```python
from build123d import *

# Parameters (mm, degrees)
F0_R      = 10
F1_DEPTH  = 10
F0_R_2    = 6
F2_DEPTH  = 20
F0_W      = 60
F0_H      = 20
F3_DEPTH  = 70
F4_R      = 16
F5_DEPTH  = 50
F6_R      = 3
F9_DEPTH  = 77.2
F10_DEPTH = 15
F11_DEPTH = 15


with BuildPart() as f1:
    # F0 (on Top) → F1 (new body)
    with BuildSketch(Plane.XY):
        with BuildLine():
            ThreePointArc((-5.564519, 60.884742), (-26.777723, 52.097945), (-35.564519, 30.884742))
            Line((-35.564519, 30.884742), (-35.564519, -9.115258))
            Line((-35.564519, -9.115258), (24.435481, -9.115258))
            Line((24.435481, -9.115258), (24.435481, 30.884742))
            ThreePointArc((24.435481, 30.884742), (15.648684, 52.097945), (-5.564519, 60.884742))
        make_face()
        with Locations((-5.564519, 30.884742)):
            Circle(F0_R, mode=Mode.SUBTRACT)
    extrude(amount=F1_DEPTH)

    # F0 (on Top) → F2 (join)
    with BuildSketch(Plane.XY):
        with Locations((-5.564519, 30.884742)):
            Circle(F0_R)
        with Locations((-5.564519, 30.884742)):
            Circle(F0_R_2, mode=Mode.SUBTRACT)
    extrude(amount=F2_DEPTH)

    # F0 (on Top) → F3 (join)
    with BuildSketch(Plane.XY):
        with Locations((-5.564519, -19.115258)):
            Rectangle(F0_W, F0_H)
    extrude(amount=F3_DEPTH)

    # F4 (on face) → F5 (join)
    with BuildSketch(Plane.XZ.offset(29.115258)):
        with Locations((-5.564519, 35)):
            Circle(F4_R)
    extrude(amount=F5_DEPTH)

    # F6
    f6_edges = [f1.edges().sort_by_distance(p)[0] for p in [
        (-21.564519, -79.115258, 35),
    ]]
    fillet(f6_edges, radius=F6_R)

    # F8 (on face) → F9 (cut)
    with BuildSketch(Plane(origin=(-35.564519, 0, 0), x_dir=(0, -1, 0), z_dir=(-1, 0, 0))):
        Polygon((19.833226, 70), (9.115258, 70), (9.115258, 30), align=None)
    extrude(amount=-F9_DEPTH, mode=Mode.SUBTRACT)

    # F8 (on face) → F10 (join)
    with BuildSketch(Plane(origin=(-35.564519, 0, 0), x_dir=(0, -1, 0), z_dir=(-1, 0, 0))):
        Polygon((19.833226, 70), (9.115258, 70), (9.115258, 30), align=None)
        Polygon((19.833226, 70), (9.115258, 30), (9.115258, 10), (-30.884742, 10), (-30.884742, 0), (29.115258, 0), (29.115258, 70), align=None)
    extrude(amount=-F10_DEPTH)

    # F7 (on face) → F11 (join)
    with BuildSketch(Plane.YZ.offset(24.435481)):
        Polygon((-9.115258, 10), (-9.115258, 30), (-19.833226, 70), (-29.115258, 70), (-29.115258, 0), (30.884742, 0), (30.884742, 10), align=None)
        Polygon((-9.115258, 30), (-9.115258, 70), (-19.833226, 70), align=None)
    extrude(amount=-F11_DEPTH)


solid = f1.part
```
Verification items for the finished model (mm, model axes). A direction names the side the tool comes from. Coordinates: 2 decimals unless noted, no trailing zeros. Order: outer loops, then holes, each group sorted by start corner. A loop starts at its lowest first (then second) coordinate and runs counter-clockwise, first axis right, second up. Notation, with made-up numbers: (63.25, 67) - (92.25, 67) arc R18 ccw to (92.25, 86) - close; hole circle Ø6 at (-27.75, 75). An arc over 180 degrees is marked (long way). Return JSON: item names as keys, results as strings.
(1) Section check B-B, the plane y = -44.5. Record the cut outline in (x, z).
Filled sheet:
{"outline": "circle Ø32 at (-5.56, 35)"}
(2) Section check A-A, the plane z = 53.5. Record the cut outline in (x, y).
Filled sheet:
{"outline": "(-35.56, -29.12) - (24.44, -29.12) - (24.44, -9.12) - (9.44, -9.12) - (9.44, -15.41) - (-20.56, -15.41) - (-20.56, -9.12) - (-35.56, -9.12) - close"}
(3) Section check C-C, the plane x = -26. Record the cut outline in (y, z).
Filled sheet:
{"outline": "(-29.12, 0) - (52.85, 0) - (52.85, 10) - (-9.12, 10) - (-9.12, 70) - (-29.12, 70) - close"}
(4) Mould release check, pull along X, two halves, no side actions. Record for faces 1 (the flat face through (-5.77, -14.4, 49.72)), 2 (the flat face through (-35.565, -12, 28)), 3 (the flat face through (-13, -29.115, 19)): pulls with the +X half, pulls with the -X half, needs draft (parallel to the pull), parting line crosses it, or undercut.
Filled sheet:
{"face 1": "undercut", "face 2": "pulls with the -X half", "face 3": "needs draft"}
(5) Access from +Z, -Z, +X, -X, +Y, -Y to the whole of each face (thin tool, end or side, straight path). Record for faces 4 (the cylindrical face through (-9.03, -52.29, 19.38)), 5 (the cylindrical face through (-7.73, 21.12, 14.93)), 6 (the flat face through (-20.565, -13, 55)), 7 (the flat face through (1, 31, 20)).
Filled sheet:
{"face 4": "-Y", "face 5": "+Z", "face 6": "+Z, +Y", "face 7": "+Z, +X, -X, +Y"}
(6) Thickness scan on line 1 along Y through (x, z) = (-5.5, 15); line 2 along Y through (x, z) = (-28, 55); line 3 along Z through (x, y) = (21.5, 28). Record the ranges inside material, lowest first.
Filled sheet:
{"line 1": "y = -29.12 to -9.12, 20.88 to 24.89, 36.88 to 40.88", "line 2": "y = -29.12 to -9.12", "line 3": "z = 0 to 10"}
(7) Go/stop test with flat-tipped pins: pin 1 (5 mm diameter, centred on x = 7.5, y = -61, fed in from -Z); pin 2 (12 mm diameter, centred on x = 14.5, z = 56, fed in from +Y); pin 3 (2 mm diameter, centred on x = 3.5, y = -64, fed in from +Z). Record where each tip stops, or that it passes through.
Filled sheet:
{"pin 1": "stops at z = 22.98", "pin 2": "stops at y = -9.12", "pin 3": "stops at z = 48.82"}
(8) Section check D-D, the plane z = 35. Record the cut outline in (x, y) (3 decimals).
Filled sheet:
{"outline": "(-35.565, -29.115) - (-21.565, -29.115) - (-21.565, -76.115) arc R3 ccw to (-18.565, -79.115) - (7.435, -79.115) arc R3 ccw to (10.435, -76.115) - (10.435, -29.115) - (24.435, -29.115) - (24.435, -9.115) - (9.435, -9.115) - (9.435, -10.455) - (-20.565, -10.455) - (-20.565, -9.115) - (-35.565, -9.115) - close"}
